from build123d import *

# Parameters (mm, degrees)
EXTRU_MINCE1_DEPTH      = 3.5
D_PLIAGE_START          = -3.5
D_PLIAGE_2_OUTLINE_W    = 2
D_PLIAGE_2_OUTLINE_H    = 7
D_PLIAGE_2_DEPTH        = 7
D_PLIAGE_2_2_OUTLINE_W  = 6.141592654
D_PLIAGE_2_2_OUTLINE_H  = 2
D_PLIAGE_2_2_DEPTH      = 7
PLIAGE_START            = -3.5
PLIAGE_2_DEPTH          = 7
PLIAGE_2_2_DEPTH        = 7
ENL_V_MAT_EXTRU_1_REACH = 11.287
ESQUISSE10_R            = 1.5
ESQUISSE11_W            = 2.5
ESQUISSE11_H            = 5
PATTE1_DEPTH            = 2
CONG_2_R                = 1
ESQUISSE13_W            = 2.5
ESQUISSE13_H            = 5
PATTE2_DEPTH            = 2
CONG_9_R                = 1
EXTRUSION2_DEPTH        = 2.5
EXTRU_MINCE2_START      = 1
ESQUISSE16_R            = 1.75
ESQUISSE16_R_2          = 1.5
EXTRU_MINCE2_DEPTH      = 1


# Read off the part's stored shape, not the designer's step: Dépliage 2, Pliage 2
# Sheet-metal steps are written as plain solids
with BuildPart() as part:
    # Esquisse1 → Extru.-Mince1 (new, symmetric)
    with BuildSketch(Plane.XY):
        Polygon((-3, 7), (-3, 0), (3, 0), (3, 7), (5, 7), (5, -2), (-5, -2), (-5, 7), align=None)
    extrude(amount=EXTRU_MINCE1_DEPTH, both=True)

    # Dépliage 2 outline → Dépliage 2 (cut)
    with BuildSketch(Plane.XY.offset(D_PLIAGE_START)):
        with Locations((4, 3.5)):
            Rectangle(D_PLIAGE_2_OUTLINE_W, D_PLIAGE_2_OUTLINE_H)
        with Locations((-4, 3.5)):
            Rectangle(D_PLIAGE_2_OUTLINE_W, D_PLIAGE_2_OUTLINE_H)
    extrude(amount=D_PLIAGE_2_DEPTH, mode=Mode.SUBTRACT)

    # D_pliage 2 2 outline → D_pliage 2 2 (add)
    with BuildSketch(Plane.XY.offset(D_PLIAGE_START)):
        with Locations((8.070796327, -1)):
            Rectangle(D_PLIAGE_2_2_OUTLINE_W, D_PLIAGE_2_2_OUTLINE_H)
        with Locations((-8.070796327, -1)):
            Rectangle(D_PLIAGE_2_2_OUTLINE_W, D_PLIAGE_2_2_OUTLINE_H)
    extrude(amount=D_PLIAGE_2_2_DEPTH)

    # Pliage 2 outline → Pliage 2 (cut)
    with BuildSketch(Plane.XY.offset(PLIAGE_START)):
        with BuildLine():
            ThreePointArc((-2, -2), (-3.732050808, -1.449489743), (-4.828427125, 0))
            Line((-4.828427125, 0), (-11.141592654, 0))
            Line((-11.141592654, 0), (-11.141592654, -2))
            Line((-11.141592654, -2), (-2, -2))
        make_face()
        with BuildLine():
            Line((11.141592654, 0), (4.828427125, 0))
            ThreePointArc((4.828427125, 0), (3.732050808, -1.449489743), (2, -2))
            Line((2, -2), (11.141592654, -2))
            Line((11.141592654, -2), (11.141592654, 0))
        make_face()
    extrude(amount=PLIAGE_2_DEPTH, mode=Mode.SUBTRACT)

    # Pliage 2 2 outline → Pliage 2 2 (add)
    with BuildSketch(Plane.XY.offset(PLIAGE_START)):
        with BuildLine():
            Line((-3, 1), (-3, 7))
            Line((-3, 7), (-5, 7))
            Line((-5, 7), (-5, 1))
            ThreePointArc((-5, 1), (-4.956795679, 0.492694064), (-4.828427125, 0))
            Line((-4.828427125, 0), (-2, 0))
            ThreePointArc((-2, 0), (-2.707106781, 0.292893219), (-3, 1))
        make_face()
        with BuildLine():
            Line((5, 7), (3, 7))
            Line((3, 7), (3, 1))
            ThreePointArc((3, 1), (2.707106781, 0.292893219), (2, 0))
            Line((2, 0), (4.828427125, 0))
            ThreePointArc((4.828427125, 0), (4.956795679, 0.492694064), (5, 1))
            Line((5, 1), (5, 7))
        make_face()
    extrude(amount=PLIAGE_2_2_DEPTH)

    # Esquisse10 → Enlèv. mat.-Extru.1 (cut, up to next)
    with BuildSketch(Plane(origin=(0, 0, 0), x_dir=(1, 0, 0), z_dir=(0, 1, 0)), mode=Mode.PRIVATE) as enl_v_mat_extru_1_sk1:
        with Locations(Location((0, 0, 0), (0, 0, 90))):
            Circle(ESQUISSE10_R)
    enl_v_mat_extru_1_tool1 = extrude(enl_v_mat_extru_1_sk1.sketch, amount=-ENL_V_MAT_EXTRU_1_REACH, mode=Mode.PRIVATE) & part.part
    add(enl_v_mat_extru_1_tool1.solids().sort_by_distance((0, 0, 0))[0], mode=Mode.SUBTRACT)

    # Esquisse11 → Patte1 (add)
    with BuildSketch(Plane.ZY.offset(5)):
        with Locations((4.75, 4)):
            Rectangle(ESQUISSE11_W, ESQUISSE11_H)
    extrude(amount=-PATTE1_DEPTH)

    # Congé2
    cong_2_edges = [part.edges().sort_by_distance(p)[0] for p in [
        (-5, 6.5, 4.75),
        (-3, 6.5, 4.75),
        (-5, 1.5, 4.75),
        (-3, 1.5, 4.75),
    ]]
    fillet(cong_2_edges, radius=CONG_2_R - 0.0001)  # a hair under: the kernel refuses the full size

    # Esquisse13 → Patte2 (add)
    with BuildSketch(Plane(origin=(5, 0, 0), x_dir=(0, 0, -1), z_dir=(1, 0, 0))):
        with Locations((-4.75, 4)):
            Rectangle(ESQUISSE13_W, ESQUISSE13_H)
    extrude(amount=-PATTE2_DEPTH)

    # Congé9
    cong_9_edges = [part.edges().sort_by_distance(p)[0] for p in [
        (5, 6.5, 4.75),
        (3, 6.5, 4.75),
        (5, 1.5, 4.75),
        (3, 1.5, 4.75),
    ]]
    fillet(cong_9_edges, radius=CONG_9_R - 0.0001)  # a hair under: the kernel refuses the full size

    # Esquisse15 → Extrusion2 (add)
    with BuildSketch(Plane.XY.offset(3.5)):
        with BuildLine():
            Line((1.5, 0), (-1.5, 0))
            ThreePointArc((-1.5, 0), (-2.5, -1), (-1.5, -2))
            Line((-1.5, -2), (1.5, -2))
            ThreePointArc((1.5, -2), (2.5, -1), (1.5, 0))
        make_face()
    extrude(amount=EXTRUSION2_DEPTH)

    # Esquisse16 → Extru.-Mince2 (add)
    with BuildSketch(Plane(origin=(0, 0, 0), x_dir=(1, 0, 0), z_dir=(0, 1, 0)).offset(EXTRU_MINCE2_START)):
        Circle(ESQUISSE16_R)
        Circle(ESQUISSE16_R_2, mode=Mode.SUBTRACT)
    extrude(amount=-EXTRU_MINCE2_DEPTH)


solid = part.part
Input: part model. Units: mm. Frame: model coordinates. A direction names the side the tool comes from. Coordinates: 2 decimals unless noted, no trailing zeros. Loops run counter-clockwise (first coordinate to the right, second up) from the corner with the lowest first, then second, coordinate; pieces in that order, holes last. Notation, with made-up numbers: (81.5, 73) -> (91.5, 73) arc R25 cw to (91.5, 98) -> close; hole circle Ø7 at (80.25, 50). An arc over 180 degrees is marked (long way). Write each question's results on one line, items separated by ' | '. Start each with the question number.
Q1. Section B-B, the plane y = 0.5. Return the cut outline in (x, z).
Q2. Section C-C, the plane x = 0. Return the cut outline in (y, z).
Q3. Section D-D, the plane y = 4.5. Return the cut outline in (x, z).
Q4. Section A-A, the plane z = 4. State how many separate pieces and enclosed holes the cut face has, plus the area to 3 significant figures.
Q5. Pin query (flat end, axial travel): pin 1 (4.5 mm diameter, centred on x = 0, z = 0, fed in from +Y). Return the tip coordinate at first contact, or that it passes through.
Q6. Reachability of faces 1 (the cylindrical face through (-3.285, 6.199, 4.768)), 2 (the flat face through (0, 0, 2)), 3 (the flat face through (3, 4, 1)), 4 (the cylindrical face through (2.5, -1, 4.7)) from +Z, -Z, +X, -X, +Y, -Y: full face, straight path, thin tool, end or side. Return the list, or none.
Q7. Ray query, line 1 (X direction, y = 5.5, z = -0.5); line 2 (Y direction, x = 2, z = 2.25); line 3 (Z direction, x = -0.75, y = -1). Return the intervals inside material, ascending. Write a range as from..to.
Found:
1) outline: (-4.96, -3.5) -> (-2.87, -3.5) -> (-2.87, 3.5) -> (-4.96, 3.5) -> close; circle Ø3.5 at (0, 0); (2.87, -3.5) -> (4.96, -3.5) -> (4.96, 3.5) -> (2.87, 3.5) -> close; hole circle Ø3 at (0, 0)
2) outline: (-2, -3.5) -> (0, -3.5) -> (0, -1.75) -> (1, -1.75) -> (1, -1.5) -> (-2, -1.5) -> close; (-2, 1.5) -> (1, 1.5) -> (1, 1.75) -> (0, 1.75) -> (0, 6) -> (-2, 6) -> close
3) outline: (-5, -3.5) -> (-3, -3.5) -> (-3, 6) -> (-5, 6) -> close; (3, -3.5) -> (5, -3.5) -> (5, 6) -> (3, 6) -> close
4) separate pieces: 3 | enclosed holes: 0 | area: 27.4 mm2
5) pin 1: y = 1
6) face 1: +Z, +Y | face 2: +Y | face 3: +Z, -Z, +Y | face 4: +Z, +X
7) line 1: -5..-3, 3..5 | line 2: -2..0 | line 3: -3.5..-1.3, 1.3..6
